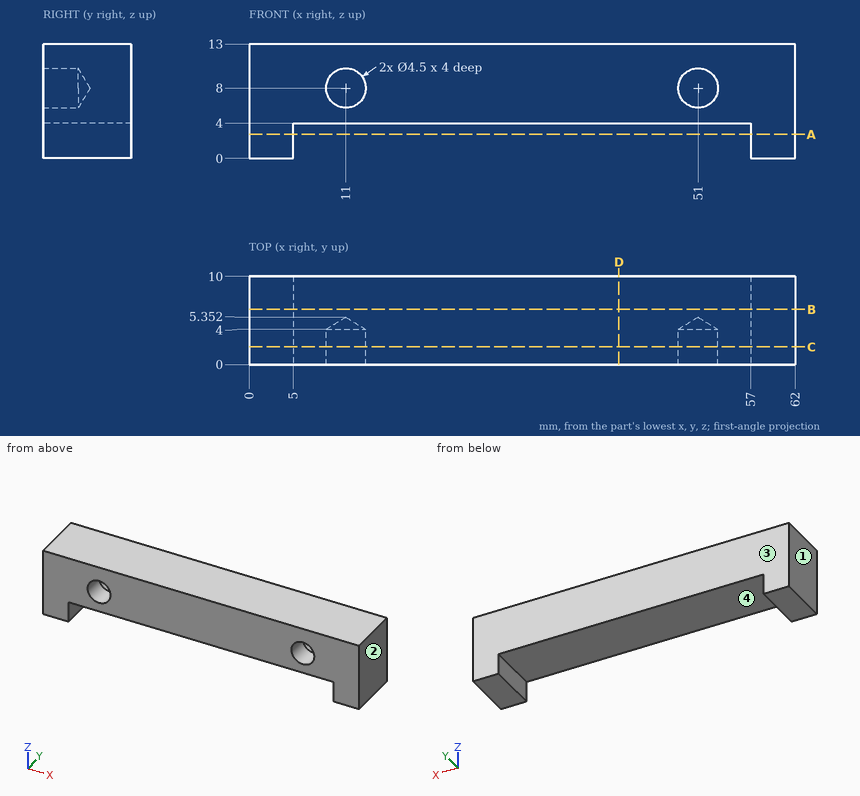
Design review of the part shown in the three views and the two pictorial views. Dimensions are in mm from the part's minimum x, y and z. Round coordinates to 2 decimals unless told otherwise and drop trailing zeros. Write each loop counter-clockwise with the first axis right and the second up, starting at its lowest first coordinate (ties: lowest second). Pieces come first, ordered by that corner, then holes.
Item 1: Draft analysis for pull direction X (two halves, no side actions). For the marked faces 1, 2, 3 and 4, state which applies: released by +X, released by -X, zero draft, split by the parting line, or undercut.
Item 2: Consider section B-B on y = 6.25. Give the boundary of the cut face in (x, z), and give its area (3 significant figures).
Item 3: Consider section A-A on z = 2.75. Give the boundary of the cut face in (x, y).
Item 4: For pin 1 Ø1 at (x, y) = (7.5, 2.5) entering from -Z, flat-tipped, find the tip position at first contact; note if it passes through.
Item 5: Consider section D-D on x = 42. Give the boundary of the cut face in (y, z).
Item 6: Consider section C-C on y = 2. Give the boundary of the cut face in (x, z), and give its area (3 significant figures).
Item 7: Wall thickness on L1, parallel to Z at x = 51, y = 0.8; L2, parallel to X at y = 6.25, z = 3.5; L3, parallel to X at y = 1.7, z = 8: over which ranges is each line inside the solid? List them lowest first.
Check values:
1. face 1: released by -X
1. face 2: released by +X
1. face 3: zero draft
1. face 4: undercut
2. outline: (0, 0) - (5, 0) - (5, 4) - (57, 4) - (57, 0) - (62, 0) - (62, 13) - (0, 13) - close
2. area: 598 mm2
3. outline: (0, 0) - (5, 0) - (5, 10) - (0, 10) - close; (57, 0) - (62, 0) - (62, 10) - (57, 10) - close
4. pin 1: stops at z = 4
5. outline: (0, 4) - (10, 4) - (10, 13) - (0, 13) - close
6. outline: (0, 0) - (5, 0) - (5, 4) - (57, 4) - (57, 0) - (62, 0) - (62, 13) - (0, 13) - close; hole circle Ø4.5 at (11, 8); hole circle Ø4.5 at (51, 8)
6. area: 566 mm2
7. L1: z = 4 to 5.75, 10.25 to 13
7. L2: x = 0 to 5, 57 to 62
7. L3: x = 0 to 8.75, 13.25 to 48.75, 53.25 to 62
